Design review of the part built by this model. Coordinates are the model's own, in mm. A direction names the side the tool comes from. Round coordinates to 2 decimals unless told otherwise and drop trailing zeros. Loops run counter-clockwise (first coordinate to the right, second up) from the corner with the lowest first, then second, coordinate; pieces in that order, holes last. Notation, with made-up numbers: (-5.75, -23.75) -> (36.25, -23.75) arc R25 ccw to (36.25, -4.75) -> close; hole circle Ø2 at (39.25, 28.5). An arc over 180 degrees is marked (long way). Use a Markdown table: item, result. Add a question column.
from build123d import *

# Parameters (mm, degrees)
SKETCH_W        = 10.7
SKETCH_H        = 24
PAD_DEPTH       = 20.7
POCKET_DEPTH    = 24.001
FILLET_R        = 6
POCKET001_DEPTH = 74.503317
SKETCH003_R     = 1.6
POCKET002_DEPTH = 4
CHAMFER_SIZE    = 3
CHAMFER001_SIZE = 3


with BuildPart() as part:
    # Sketch → Pad (new body)
    with BuildSketch(Plane.XY):
        Rectangle(SKETCH_W, SKETCH_H)
    extrude(amount=PAD_DEPTH)

    # Sketch001 (on Face3 of Pad) → Pocket (cut, through all)
    with BuildSketch(Plane.XZ.offset(12)):
        Polygon((-0.95, 20.7), (0.1, 7.6), (-5.35, 7.6), (-5.35, 20.7), align=None)
    extrude(amount=-POCKET_DEPTH, mode=Mode.SUBTRACT)

    # Fillet
    fillet_edges = [part.edges().sort_by_distance(p)[0] for p in [
        (5.35, 0, 0),
    ]]
    fillet(fillet_edges, radius=FILLET_R)

    # Sketch002 (on Face6 of Fillet) → Pocket001 (cut, through all)
    with BuildSketch(Plane.XY.offset(7.6)):
        Polygon((-5.35, 12), (-3.4, 9.8), (-3.4, 4.5), (-5.35, 3.73), align=None)
    pocket001 = extrude(amount=-POCKET001_DEPTH, mode=Mode.SUBTRACT)

    # Mirrored: Pocket001 across Sketch002 H_Axis
    add(pocket001.mirror(Plane(origin=(0, 0, 7.6), x_dir=(0, 0, 1), z_dir=(0, 1, 0))), mode=Mode.SUBTRACT)

    # Sketch003 (on Face9 of Mirrored) → Pocket002 (cut)
    with BuildSketch(Plane(origin=(-3.4, 0, 0), x_dir=(0, -1, 0), z_dir=(-1, 0, 0))):
        with Locations((-7, 3.8)):
            Circle(SKETCH003_R)
    pocket002 = extrude(amount=-POCKET002_DEPTH, mode=Mode.SUBTRACT)

    # Mirrored001: Pocket002 across Sketch003 V_Axis
    add(pocket002.mirror(Plane(origin=(-3.4, 0, 0), x_dir=(-1, 0, 0), z_dir=(0, -1, 0))), mode=Mode.SUBTRACT)

    # Chamfer
    chamfer_edges = [part.edges().sort_by_distance(p)[0] for p in [
        (5.35, -12, 13.35),
    ]]
    chamfer(chamfer_edges, length=CHAMFER_SIZE)

    # Chamfer001
    chamfer001_edges = [part.edges().sort_by_distance(p)[0] for p in [
        (5.35, 12, 13.35),
    ]]
    chamfer(chamfer001_edges, length=CHAMFER001_SIZE)


solid = part.part
1. Consider section A-A on x = -2. State the section outline as (y, z) points.
2. Mouldability with a two-part tool opening along Z and no side actions: class faces 5 (the face through (2, -11, 3)), 6 (the face through (0.2, -12, 9.8)), 7 (the face through (-1.43, 7.35, 2.24)) as +Z half, -Z half, draft (parallel to the pull), parting line (faces both ways), or undercut.
3. Consider section C-C on x = -3.75. State the section outline as (y, z) points, plus the area to 3 significant figures.
4. To check wall thickness, follow probe 1 along Z at (x, y) = (-2.2, 7); probe 2 along Z at (x, y) = (-2.75, -7.75); probe 3 along Z at (x, y) = (-2.25, 4). State the ranges of each line that lie inside material, in increasing order. Write a range as from..to.
5. For faces 1 (the face through (0.6, 7, 4)), 2 (the face through (-3, -11, 2)), 3 (the face through (-4.389, 10.915, 5.003)), 4 (the face through (-2, 0, 7.6)), list the 3-axis set-ups (+Z, -Z, +X, -X, +Y, -Y) from which the entire face can be reached by the end or side of a thin tool; tool diameter is ignored.
6. Consider section D-D on y = -1.75. State the section outline as (x, z) points, plus the area to 3 significant figures.
7. Consider section B-B on y = -7. State the section outline as (x, z) points, plus the area to 3 significant figures.
8. Insertion check: P1, Ø6, axis at y = -8, z = 2, coming from the -X side; P2, Ø4, axis at y = -5, z = 16, coming from the -X side; P3, Ø2, axis at x = -1, z = 15.5, coming from the +Y side; P4, Ø3, axis at y = -2.5, z = 10, coming from the -X side. Each pin has a flat end and moves straight along its axis. Give the tip position at first contact, or say it passes through.
Verdict:
| question | item | result |
|---|---|---|
| 1 | outline | (-12, 3) -> (-9, 0) -> (9, 0) -> (12, 3) -> (12, 7.6) -> (-12, 7.6) -> close; hole circle Ø3.2 at (-7, 3.8); hole circle Ø3.2 at (7, 3.8) |
| 2 | face 5 | -Z half |
| 2 | face 6 | draft |
| 2 | face 7 | undercut |
| 3 | outline | (-12, 3) -> (-10.19, 1.19) -> (-10.19, 7.6) -> (-12, 7.6) -> close; (-4.36, 0) -> (4.36, 0) -> (4.36, 7.6) -> (-4.36, 7.6) -> close; (10.19, 1.19) -> (12, 3) -> (12, 7.6) -> (10.19, 7.6) -> close |
| 3 | area | 86.2 mm² |
| 4 | probe 1 | z = 0..2.2, 5.4..7.6 |
| 4 | probe 2 | z = 0..2.39, 5.21..7.6 |
| 4 | probe 3 | z = 0..7.6 |
| 5 | face 1 | -X |
| 5 | face 2 | -Z, +X, -X, -Y |
| 5 | face 3 | +Z, -Z, -X |
| 5 | face 4 | -X, +Y, -Y |
| 6 | outline | (-5.35, 0) -> (-0.65, 0) arc R6 ccw to (5.35, 6) -> (5.35, 20.7) -> (-0.95, 20.7) -> (0.1, 7.6) -> (-5.35, 7.6) -> close |
| 6 | area | 149 mm² |
| 7 | outline | (-3.4, 0) -> (-0.65, 0) arc R6 ccw to (5.35, 6) -> (5.35, 20.7) -> (-0.95, 20.7) -> (0.1, 7.6) -> (-3.4, 7.6) -> (-3.4, 5.4) -> (0.6, 5.4) -> (0.6, 2.2) -> (-3.4, 2.2) -> close |
| 7 | area | 122 mm² |
| 8 | P1 | stops at x = -4.46 |
| 8 | P2 | stops at x = -0.73 |
| 8 | P3 | stops at y = 12 |
| 8 | P4 | stops at x = -0.21 |
